The listing builds one solid part. Answer for the finished solid, in the listing's coordinates (mm). A direction names the side the tool comes from. Give positions to 0.01 mm unless a question says otherwise; leave off trailing zeros. Write each loop counter-clockwise with the first axis right and the second up, starting at its lowest first coordinate (ties: lowest second). Pieces come first, ordered by that corner, then holes. Notation, with made-up numbers: (36, -4) - (81, -4) arc R12 cw to (81, 5) - close; hole circle Ø8 at (-5, 8.25). An arc over 180 degrees is marked (long way). Use a Markdown table: item, result. Add a question column.
from build123d import *

# Parameters (mm, degrees)
SKETCH_1_W                         = 148
SKETCH_1_H                         = 90
SM_BASE_FLANGE_1_DEPTH             = 0.7
SM_EDGE_FLANGE_1_STRIP_W           = 3.2
SM_EDGE_FLANGE_1_STRIP_H           = 0.7
SM_EDGE_FLANGE_1_STRIP_CUT_DEPTH   = 90
SM_EDGE_FLANGE_1_STRIP_2_W         = 3.2
SM_EDGE_FLANGE_1_STRIP_2_H         = 0.7
SM_EDGE_FLANGE_1_STRIP_CUT_2_DEPTH = 90
SM_EDGE_FLANGE_1_DEPTH             = 90
SM_EDGE_FLANGE_1_PROFILE_W         = 90
SM_EDGE_FLANGE_1_PROFILE_H         = 11.1
SM_EDGE_FLANGE_1_PROFILE_R         = 3
SM_EDGE_FLANGE_1_FLAT_DEPTH        = 0.7
SM_EDGE_FLANGE_1_BEND_DEPTH        = 90
FILLET_2_R                         = 5
CUT_EXTRUDE_START                  = -10
SKETCH_15_R                        = 3
CUT_EXTRUDE_1_DEPTH                = 10


# Sheet-metal steps are written as plain solids
with BuildPart() as part:
    # Sketch 1 → 基体-法兰1 (new body)
    with BuildSketch(Plane(origin=(0, 0, 0), x_dir=(1, 0, 0), z_dir=(0, 1, 0))):
        Rectangle(SKETCH_1_W, SKETCH_1_H)
        with BuildLine():
            Line((-46, 37), (-38, 37))
            ThreePointArc((-38, 37), (-35, 34), (-38, 31))
            Line((-38, 31), (-46, 31))
            ThreePointArc((-46, 31), (-49, 34), (-46, 37))
        make_face(mode=Mode.SUBTRACT)
        with BuildLine():
            Line((38, 37), (46, 37))
            ThreePointArc((46, 37), (49, 34), (46, 31))
            Line((46, 31), (38, 31))
            ThreePointArc((38, 31), (35, 34), (38, 37))
        make_face(mode=Mode.SUBTRACT)
    extrude(amount=-SM_BASE_FLANGE_1_DEPTH)

    # 边线-法兰1 strip (across the edge) → 边线-法兰1 strip cut (cut)
    with BuildSketch(Plane(origin=(74, -0.7, -45), x_dir=(-1, 0, 0), z_dir=(0, 0, 1))):
        with Locations((-0.7, -0.35)):
            Rectangle(SM_EDGE_FLANGE_1_STRIP_W, SM_EDGE_FLANGE_1_STRIP_H)
    extrude(amount=SM_EDGE_FLANGE_1_STRIP_CUT_DEPTH, mode=Mode.SUBTRACT)

    # 边线-法兰1 strip 2 (across the edge) → 边线-法兰1 strip cut 2 (cut)
    with BuildSketch(Plane(origin=(-74, -0.7, 45), x_dir=(1, 0, 0), z_dir=(0, 0, -1))):
        with Locations((-0.7, -0.35)):
            Rectangle(SM_EDGE_FLANGE_1_STRIP_2_W, SM_EDGE_FLANGE_1_STRIP_2_H)
    extrude(amount=SM_EDGE_FLANGE_1_STRIP_CUT_2_DEPTH, mode=Mode.SUBTRACT)

    # 边线-法兰1 bend section (across the edge) → 边线-法兰1 (add)
    with BuildSketch(Plane(origin=(74, -0.7, -45), x_dir=(-1, 0, 0), z_dir=(0, 0, 1))):
        with BuildLine():
            Line((0, 0.2), (0.7, 0.2))
            ThreePointArc((0.7, 0.2), (0.758578644, 0.058578644), (0.9, 0))
            Line((0.9, 0), (0.9, -0.7))
            ThreePointArc((0.9, -0.7), (0.263603897, -0.436396103), (0, 0.2))
        make_face()
    extrude(amount=SM_EDGE_FLANGE_1_DEPTH)

    # 边线-法兰1 profile (on flange) → 边线-法兰1 flat (add)
    with BuildSketch(Plane(origin=(74, -0.7, 0), x_dir=(0, 0, 1), z_dir=(1, 0, 0))):
        with Locations((0, 5.75)):
            Rectangle(SM_EDGE_FLANGE_1_PROFILE_W, SM_EDGE_FLANGE_1_PROFILE_H)
        with Locations((17, 6.8)):
            Circle(SM_EDGE_FLANGE_1_PROFILE_R, mode=Mode.SUBTRACT)
        with Locations((27, 6.8)):
            Circle(SM_EDGE_FLANGE_1_PROFILE_R, mode=Mode.SUBTRACT)
        with Locations((-33, 6.8)):
            Circle(SM_EDGE_FLANGE_1_PROFILE_R, mode=Mode.SUBTRACT)
    extrude(amount=-SM_EDGE_FLANGE_1_FLAT_DEPTH)

    # 边线-法兰1 section (across the edge) → 边线-法兰1 bend (add)
    with BuildSketch(Plane(origin=(-74, -0.7, 45), x_dir=(1, 0, 0), z_dir=(0, 0, -1))):
        with BuildLine():
            Line((0, 0.2), (0, 11.3))
            Line((0, 11.3), (0.7, 11.3))
            Line((0.7, 11.3), (0.7, 0.2))
            ThreePointArc((0.7, 0.2), (0.758578644, 0.058578644), (0.9, 0))
            Line((0.9, 0), (0.9, -0.7))
            ThreePointArc((0.9, -0.7), (0.263603897, -0.436396103), (0, 0.2))
        make_face()
    extrude(amount=SM_EDGE_FLANGE_1_BEND_DEPTH)

    # 圆角2
    fillet_2_edges = [part.edges().sort_by_distance(p)[0] for p in [
        (-73.65, -12, 45),
        (-73.65, -12, -45),
        (73.65, -12, -45),
        (73.65, -12, 45),
    ]]
    fillet(fillet_2_edges, radius=FILLET_2_R)

    # 草图15 → 切除-拉伸1 (cut)
    with BuildSketch(Plane.ZY.offset(74).offset(CUT_EXTRUDE_START)):
        with Locations(Location((-33, -7.5, 0), (0, 0, 270))):
            Circle(SKETCH_15_R)
        with Locations(Location((17, -7.5, 0), (0, 0, 270))):
            Circle(SKETCH_15_R)
        with Locations(Location((27, -7.5, 0), (0, 0, 270))):
            Circle(SKETCH_15_R)
    extrude(amount=CUT_EXTRUDE_1_DEPTH, mode=Mode.SUBTRACT)


solid = part.part
1. The part is cut by section B-B (z = 18.5). Give the vertices of the cut face in (x, y).
2. The part is cut by section C-C (z = -8). Give the vertices of the cut face in (x, y), and give its area (3 significant figures).
3. The part is cut by section A-A (x = -36.5). Give the vertices of the cut face in (y, z), and give its area (3 significant figures).
4. The part is cut by section D-D (z = -33). Give the vertices of the cut face in (x, y).
5. Consider L1, parallel to Z at x = 73.65, y = -7.5; L2, parallel to X at y = -5.75, z = 39.5; L3, parallel to Y at x = -73.7, z = -33. Determine where each line is inside the solid, lowest interval first. Write a range as [from, to].
6. Given P1, Ø10, axis at x = -44, z = -26, coming from the +Y side; P2, Ø3, axis at x = 42.5, z = 23.5, coming from the -Y side, each flat-ended and moving along its own axis, determine where each tip first touches the part or whether it passes through.
7. Which of the six approach directions +Z, -Z, +X, -X, +Y, -Y give full straight-line access (tool end or side, diameter ignored) to faces 1 (the cylindrical face through (49, -0.3, -34.1)), 2 (the cylindrical face through (-73.65, -10.57, 43.5)), 3 (the flat face through (-1, -0.7, -1))?
8. For a pull along Z with two mould halves and no side action, classify faces 4 (the flat face through (73.3, -7, -1)), 5 (the cylindrical face through (73.7, -7.6, 24)), 6 (the cylindrical face through (73.65, -10.5, 43.57)), 7 (the cylindrical face through (35, -0.3, -33.9)) as released by +Z, released by -Z, zero draft, split by the parting line, or undercut.
Check values:
| question | item | result |
|---|---|---|
| 1 | outline | (-74, -12) - (-73.3, -12) - (-73.3, -10.1) - (-74, -10.1) - close; (-74, -4.9) - (-73.3, -4.9) - (-73.3, -0.9) arc R0.2 cw to (-73.1, -0.7) - (73.1, -0.7) arc R0.2 cw to (73.3, -0.9) - (73.3, -4.9) - (74, -4.9) - (74, -0.9) arc R0.9 ccw to (73.1, 0) - (-73.1, 0) arc R0.9 ccw to (-74, -0.9) - close; (73.3, -12) - (74, -12) - (74, -10.1) - (73.3, -10.1) - close |
| 2 | outline | (-74, -12) - (-73.3, -12) - (-73.3, -0.9) arc R0.2 cw to (-73.1, -0.7) - (73.1, -0.7) arc R0.2 cw to (73.3, -0.9) - (73.3, -12) - (74, -12) - (74, -0.9) arc R0.9 ccw to (73.1, 0) - (-73.1, 0) arc R0.9 ccw to (-74, -0.9) - close |
| 2 | area | 119 mm2 |
| 3 | outline | (-0.7, -45) - (0, -45) - (0, -36.6) - (-0.7, -36.6) - close; (-0.7, -31.4) - (0, -31.4) - (0, 45) - (-0.7, 45) - close |
| 3 | area | 59.4 mm2 |
| 4 | outline | (-74, -12) - (-73.3, -12) - (-73.3, -10.5) - (-74, -10.5) - close; (-74, -4.5) - (-73.3, -4.5) - (-73.3, -0.9) arc R0.2 cw to (-73.1, -0.7) - (-48.83, -0.7) - (-48.83, 0) - (-73.1, 0) arc R0.9 ccw to (-74, -0.9) - close; (-35.17, -0.7) - (35.17, -0.7) - (35.17, 0) - (-35.17, 0) - close; (48.83, -0.7) - (73.1, -0.7) arc R0.2 cw to (73.3, -0.9) - (73.3, -4.5) - (74, -4.5) - (74, -0.9) arc R0.9 ccw to (73.1, 0) - (48.83, 0) - close; (73.3, -12) - (74, -12) - (74, -10.5) - (73.3, -10.5) - close |
| 5 | L1 | z = [-44.97, -36], [-30, 14], [20, 24], [30, 44.97] |
| 5 | L2 | x = [-74, -73.3], [73.3, 74] |
| 5 | L3 | y = [-12, -10.5], [-4.5, -0.23] |
| 6 | P1 | stops at y = 0 |
| 6 | P2 | stops at y = -0.7 |
| 7 | face 1 | +Y, -Y |
| 7 | face 2 | +Z, +X, -X, -Y |
| 7 | face 3 | +Z, -Z, -Y |
| 8 | face 4 | zero draft |
| 8 | face 5 | undercut |
| 8 | face 6 | released by +Z |
| 8 | face 7 | undercut |
